Design review of the part built by this model. Coordinates are the model's own, in mm. A direction names the side the tool comes from. Coordinates: 2 decimals unless noted, no trailing zeros. Loops run counter-clockwise (first coordinate to the right, second up) from the corner with the lowest first, then second, coordinate; pieces in that order, holes last. Notation, with made-up numbers: (84, 23.5) -> (105, 23.5) arc R12 cw to (105, 39.5) -> close; hole circle Ø8 at (84.25, -11.75). An arc over 180 degrees is marked (long way). Answer as a JSON object with one key per item and string values.
```python
from build123d import *

# Parameters (mm, degrees)
F0_W     = 150
F0_H     = 20
F1_DEPTH = 15
F2_W     = 150
F2_H     = 15
F3_DEPTH = 13
F4_R     = 2
F5_DEPTH = 2.5
F6_R     = 2
F7_R     = 1


with BuildPart() as f1:
    # F0 (on Top) → F1 (new body)
    with BuildSketch(Plane.XY):
        with Locations((1.380986, -6.045858)):
            Rectangle(F0_W, F0_H)
    extrude(amount=F1_DEPTH)

    # F2 (on face) → F3 (cut)
    with BuildSketch(Plane.XY.offset(15)):
        with Locations((1.380986, -6.045858)):
            Rectangle(F2_W, F2_H)
    extrude(amount=-F3_DEPTH, mode=Mode.SUBTRACT)

    # F4 (on face) → F5 (cut)
    with BuildSketch(Plane(origin=(0, 3.954142, 0), x_dir=(-1, 0, 0), z_dir=(0, 1, 0))):
        with Locations((-38.880986, 10)):
            Circle(F4_R)
        with Locations((-1.380986, 10)):
            Circle(F4_R)
        with Locations((36.119014, 10)):
            Circle(F4_R)
    extrude(amount=-F5_DEPTH, mode=Mode.SUBTRACT)

    # F6
    f6_edges = [f1.edges().sort_by_distance(p)[0] for p in [
        (1.380986, -16.045858, 0),
        (1.380986, 3.954142, 0),
    ]]
    fillet(f6_edges, radius=F6_R)

    # F7
    f7_edges = [f1.edges().sort_by_distance(p)[0] for p in [
        (1.380986, -13.545858, 2),
        (1.380986, 1.454142, 2),
    ]]
    fillet(f7_edges, radius=F7_R)


solid = f1.part
```
1) The part is to be moulded in two halves that separate along X. For faces 4 (the flat face through (-73.619, -7, 1)), 5 (the cylindrical face through (1.641, 2.722, 11.983)), 6 (the flat face through (0, 1.454, 8)), say which applies: pulls with the +X half, pulls with the -X half, needs draft (parallel to the pull), parting line crosses it, or undercut.
Completed:
{"face 4": "pulls with the -X half", "face 5": "undercut", "face 6": "needs draft"}
2) For faces 1 (the cylindrical face through (40.88, 2.72, 10.09)), 2 (the flat face through (0, -6, 2)), 3 (the flat face through (0, -15, 15)), list the 3-axis set-ups (+Z, -Z, +X, -X, +Y, -Y) from which the entire face can be reached by the end or side of a thin tool; tool diameter is ignored.
Completed:
{"face 1": "+Y", "face 2": "+Z, +X, -X", "face 3": "+Z, +X, -X, +Y, -Y"}
3) Clearance check with flat-ended pins moving along their axes: pin 1 Ø2 at (x, y) = (43.5, -1) entering from +Z; pin 2 Ø2.5 at (x, z) = (1.38, 10) entering from +Y; pin 3 Ø5 at (y, z) = (-10, 6) entering from +X. State where each tip first meets the part, or that it passes through.
Completed:
{"pin 1": "z = 2", "pin 2": "y = -13.55", "pin 3": "through"}
4) Wall thickness on probe 1 along Y at (x, z) = (-58, 11.5); probe 2 along Z at (x, y) = (45, -1); probe 3 along Y at (x, z) = (3, 10): over which ranges is each line inside the solid? List them lowest first.
Completed:
{"probe 1": "-16.05 to -13.55, 1.45 to 3.95", "probe 2": "0 to 2", "probe 3": "-16.05 to -13.55"}
5) Add section C-C, the plane y = -10. Give the boundary of the cut face in (x, z).
Completed:
{"outline": "(-73.62, 0) -> (76.38, 0) -> (76.38, 2) -> (-73.62, 2) -> close"}
6) Add section A-A, the plane z = 10. Give the boundary of the cut face in (x, y), and give its area (3 significant figures).
Completed:
{"outline": "(-73.62, -16.05) -> (76.38, -16.05) -> (76.38, -13.55) -> (-73.62, -13.55) -> close; (-73.62, 1.45) -> (-38.12, 1.45) -> (-38.12, 3.95) -> (-73.62, 3.95) -> close; (-34.12, 1.45) -> (-0.62, 1.45) -> (-0.62, 3.95) -> (-34.12, 3.95) -> close; (3.38, 1.45) -> (36.88, 1.45) -> (36.88, 3.95) -> (3.38, 3.95) -> close; (40.88, 1.45) -> (76.38, 1.45) -> (76.38, 3.95) -> (40.88, 3.95) -> close", "area": "720 mm²"}
7) Add section B-B, the plane x = -14. Give the boundary of the cut face in (y, z).
Completed:
{"outline": "(-16.05, 2) arc R2 ccw to (-14.05, 0) -> (1.95, 0) arc R2 ccw to (3.95, 2) -> (3.95, 15) -> (1.45, 15) -> (1.45, 3) arc R1 cw to (0.45, 2) -> (-12.55, 2) arc R1 cw to (-13.55, 3) -> (-13.55, 15) -> (-16.05, 15) -> close"}
